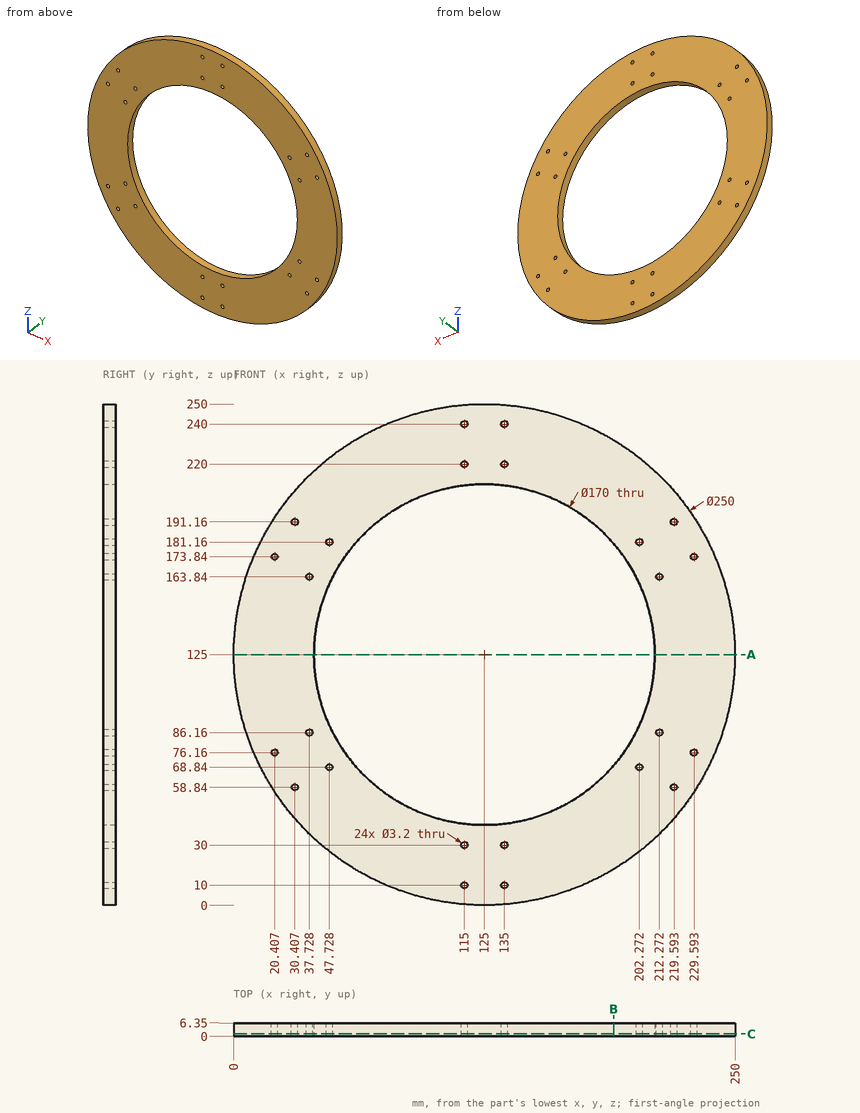
Study the drawing (mm; zero at the part's minimum x, y, z) and answer. Give positions to 0.01 mm unless a question says otherwise; leave off trailing zeros. Order: outer loops, then holes, each group sorted by start corner. A loop starts at its lowest first (then second) coordinate and runs counter-clockwise, first axis right, second up. Notation, with made-up numbers: (42.5, 73) - (95.5, 73) arc R16 cw to (95.5, 91) - close; hole circle Ø11 at (-12.5, 29.5). An arc over 180 degrees is marked (long way). Answer as CSV lines item,"result". Start each with the question number.
Q1. Find the intervals of material crossed by L1, parallel to Z at x = 135, y = 5; L2, parallel to X at y = 3.5, z = 125; L3, parallel to X at y = 5, z = 181.5 (1 decimal), in increasing order. Write a range as [from, to].
Q2. The part is cut by section A-A (z = 125). Write down the section's boundary in (x, y).
Q3. The part is cut by section C-C (y = 1). Give the number of separate pieces and of enclosed holes in the cut face, then the cut area to 3 significant figures.
Q4. Given pin 1 Ø4 at (x, z) = (135, 240) entering from +Y; pin 2 Ø1.5 at (y, z) = (3, 61.5) entering from +X; pin 3 Ø1.5 at (x, y) = (217.5, 4.5) entering from +Z (1 decimal); pin 4 Ø2 at (y, z) = (2, 48.5) entering from -X, each flat-ended and moving along its own axis, determine where each tip first touches the part or whether it passes through.
Q5. The part is cut by section B-B (x = 189.5). Write down the section's boundary in (y, z), then the cut area to 3 significant figures.
Check result:
1,L1,"z = [0.4, 8.4], [11.6, 28.4], [31.6, 40.59], [209.41, 218.4], [221.6, 238.4], [241.6, 249.6]"
1,L2,"x = [0, 40], [210, 250]"
1,L3,"x = [13.5, 46.2], [49.3, 61.5], [188.5, 200.7], [203.8, 236.5]"
2,outline,"(0, 0) - (40, 0) - (40, 6.35) - (0, 6.35) - close; (210, 0) - (250, 0) - (250, 6.35) - (210, 6.35) - close"
3,separate pieces,"1"
3,enclosed holes,"25"
3,area,"26,200 mm²"
4,pin 1,"stops at y = 6.35"
4,pin 2,"stops at x = 233.11"
4,pin 3,"stops at z = 209.9"
4,pin 4,"stops at x = 25.38"
5,outline,"(0, 17.93) - (6.35, 17.93) - (6.35, 69.64) - (0, 69.64) - close; (0, 180.36) - (6.35, 180.36) - (6.35, 232.07) - (0, 232.07) - close"
5,area,"657 mm²"
